Autodesk Inventor part; units mm, degrees
ref_plane "YZ Plane" through (0, 0, 0) normal (1, 0, 0) x (0, 1, 0)
ref_plane "XZ Plane" through (0, 0, 0) normal (0, 1, 0) x (-1, 0, 0)
ref_plane "XY Plane" through (0, 0, 0) normal (0, 0, 1) x (1, 0, 0)
sketch "Sketch1" plane through (0, 0, 0) normal (1, 0, 0) x (0, 1, 0)
  line L0 (82.3549, 27.169) -> (-47.6451, 27.169)
  line L1 (-47.6451, 27.169) -> (-47.6451, -28.031)
  line L2 (-47.6451, -28.031) -> (82.3549, -28.031)
  line L3 (82.3549, -28.031) -> (82.3549, 27.169)
  point P0 (0, 0)
  dimension "d0" = 130
  dimension "d1" = 55.2
extrude "Extrusion1" add sketch "Sketch1" along normal blind 5
sketch "Sketch3" plane through (5, 0, 0) normal (1, 0, 0) x (0, 0, -1)
  line L0 (-27.169, -47.6451) -> (28.031, -47.6451)
  line L1 (28.031, -47.6451) -> (5.831, -47.6451)
  line L2 (5.831, -47.6451) -> (5.831, -37.6451)
  point P0 (0, 0)
  dimension "d12" = 22.2
  dimension "d13" = 10
hole "Hole2" at (5, -37.6451, -5.831) direction (-1, 0, 0) diameter 3.2 end through all
sketch "Sketch13" plane through (5, 0, 0) normal (1, 0, 0) x (0, 0, -1)
  line L0 (-27.169, -47.6451) -> (28.031, -47.6451)
  line L1 (28.031, 82.3549) -> (-27.169, 82.3549)
  line L2 (28.031, -47.6451) -> (26.531, -47.6451)
  line L3 (26.531, -47.6451) -> (26.531, 82.3549)
  line L4 (26.531, 82.3549) -> (28.031, 82.3549)
  line L5 (28.031, 82.3549) -> (28.031, -47.6451)
  line L6 (-27.169, 82.3549) -> (-27.169, -47.6451)
  line L7 (28.031, 82.3549) -> (-27.169, 82.3549)
  line L8 (-27.169, -47.6451) -> (-25.669, -47.6451)
  line L9 (-25.669, -47.6451) -> (-25.669, 82.3549)
  line L10 (-25.669, 82.3549) -> (-27.169, 82.3549)
  line L11 (-27.169, 82.3549) -> (-27.169, -47.6451)
  line L12 (28.031, -47.6451) -> (-27.169, -47.6451)
  line L13 (-27.169, -47.6451) -> (-27.169, -45.6451)
  line L14 (-27.169, -45.6451) -> (28.031, -45.6451)
  line L15 (28.031, -45.6451) -> (28.031, -47.6451)
  point P0 (0, 0)
  point P1 (10.031, 62.3549)
  point P2 (-5.969, 62.3549)
  point P3 (26.531, -45.6451)
  point P4 (-25.669, -45.6451)
  point P5 (18.031, 62.3549)
  dimension "d42" = 1.5
  dimension "d43" = 1.5
  dimension "d44" = 2
extrude "Extrusion7" add sketch "Sketch13" along normal blind 6 contours L6 L14 L9 L0 | L9 L14 L3 L0 | L6 L1 L9 L14 | L3 L14 L5 L0 | L3 L1 L5 L14
sketch "Sketch18" plane through (5, 0, 0) normal (1, 0, 0) x (0, 0, -1)
  line L0 (-3.669, 82.3549) -> (4.531, 82.3549)
  line L1 (26.531, 82.3549) -> (-25.669, 82.3549)
  line L2 (4.531, 82.3549) -> (4.8312, 82.3549)
  line L3 (-3.669, 82.3549) -> (-3.969, 82.3549)
  line L4 (-3.969, 82.3549) -> (-3.969, 78.5449)
  line L5 (4.8312, 82.3549) -> (4.8312, 78.5449)
  line L6 (4.8312, 78.5449) -> (11.7812, 78.5449)
  line L7 (-3.969, 78.5449) -> (-10.919, 78.5449)
  line L8 (-10.919, 78.5449) -> (-10.919, 73.5449)
  line L9 (11.7812, 78.5449) -> (11.7812, 73.5449)
  line L10 (-10.919, 73.5449) -> (0, 73.5449)
  line L11 (0, 73.5449) -> (11.7812, 73.5449)
  point P0 (0, 0)
  point P1 (11.531, 82.3549)
  dimension "d78" = 0.3
  dimension "d79" = 3.81
  dimension "d81" = 3.81
  dimension "d83" = 6.95
  dimension "d85" = 6.95
  dimension "d86" = 5
  dimension "d87" = 5
extrude "Extrusion10" cut sketch "Sketch18" against normal blind 7.9375
properties part number "pumpholderinverseproto1"
For this review, take the finished solid that the model builds, in its own axes (mm). A direction names the side the tool comes from. Coordinates: 2 decimals unless noted, no trailing zeros. Loops run counter-clockwise (first coordinate to the right, second up) from the corner with the lowest first, then second, coordinate; pieces in that order, holes last. Notation, with made-up numbers: (70.25, 46.5) - (118.25, 46.5) arc R10 cw to (118.25, 60.5) - close; hole circle Ø2 at (28.25, 34.5). An arc over 180 degrees is marked (long way). Return JSON: item names as keys, results as strings.
Item 1: Take a section at C-C (y = 25). Give the boundary of the cut face in (x, z).
Determined:
{"outline": "(0, -28.03) - (11, -28.03) - (11, -26.53) - (5, -26.53) - (5, 25.67) - (11, 25.67) - (11, 27.17) - (0, 27.17) - close"}
Item 2: For line 1 (Z direction, x = 8.25, y = -19); line 2 (X direction, y = 54, z = -9); line 3 (Y direction, x = 9.25, z = -19), list the stretches that pass through material, from the lowest coordinate up.
Determined:
{"line 1": "z = -28.03 to -26.53, 25.67 to 27.17", "line 2": "x = 0 to 5", "line 3": "y = -47.65 to -45.65"}
Item 3: For faces 4 (the flat face through (3, 80, -4.831)), 5 (the flat face through (5, -47.645, 0)), 6 (the flat face through (3, 76, -11.781)), 7 (the flat face through (8, 17, 25.669)), list the 3-axis set-ups (+Z, -Z, +X, -X, +Y, -Y) from which the entire face can be reached by the end or side of a thin tool; tool diameter is ignored.
Determined:
{"face 4": "+X, -X, +Y", "face 5": "+Z, -Z, +X, -X, -Y", "face 6": "+X, -X", "face 7": "+X, +Y"}
Item 4: Mouldability with a two-part tool opening along Z and no side actions: class faces 1 (the flat face through (5, 16, -28.031)), 2 (the flat face through (8, -45.645, 0)), 3 (the flat face through (3, 82.355, -17)) as pulls with the +Z half, pulls with the -Z half, needs draft (parallel to the pull), parting line crosses it, or undercut.
Determined:
{"face 1": "pulls with the -Z half", "face 2": "undercut", "face 3": "needs draft"}
Item 5: Insertion check: pin 1 (3 mm diameter, centred on y = -37.65, z = -5.83, fed in from +X); pin 2 (1.5 mm diameter, centred on x = 9.5, z = 7, fed in from +Y). Each pin has a flat end and moves straight along its axis. Give the tip position at first contact, or say it passes through.
Determined:
{"pin 1": "passes through", "pin 2": "stops at y = -45.65"}
Item 6: Take a section at D-D (z = 2). Give the boundary of the cut face in (x, y).
Determined:
{"outline": "(0, -47.65) - (11, -47.65) - (11, -45.65) - (5, -45.65) - (5, 73.54) - (0, 73.54) - close"}
Item 7: Take a section at B-B (z = 22). Give the boundary of the cut face in (x, y), then the cut area to 3 significant figures.
Determined:
{"outline": "(0, -47.65) - (11, -47.65) - (11, -45.65) - (5, -45.65) - (5, 82.35) - (0, 82.35) - close", "area": "662 mm2"}
Item 8: Take a section at A-A (x = 7). Give the boundary of the cut face in (y, z).
Determined:
{"outline": "(-47.65, -28.03) - (82.35, -28.03) - (82.35, -26.53) - (-45.65, -26.53) - (-45.65, 25.67) - (82.35, 25.67) - (82.35, 27.17) - (-47.65, 27.17) - close"}
